Design review of the part built by this model. Coordinates are the model's own, in mm. Face numbers are marked on the shaded views. A direction names the side the tool comes from. Coordinates: 2 decimals unless noted, no trailing zeros. Write each loop counter-clockwise with the first axis right and the second up, starting at its lowest first coordinate (ties: lowest second). Pieces come first, ordered by that corner, then holes. Notation, with made-up numbers: (-26, 66.5) - (12, 66.5) arc R5 cw to (12, 75.5) - close; hole circle Ø7 at (68.25, 77). An arc over 180 degrees is marked (long way). One line per item, written item: value.
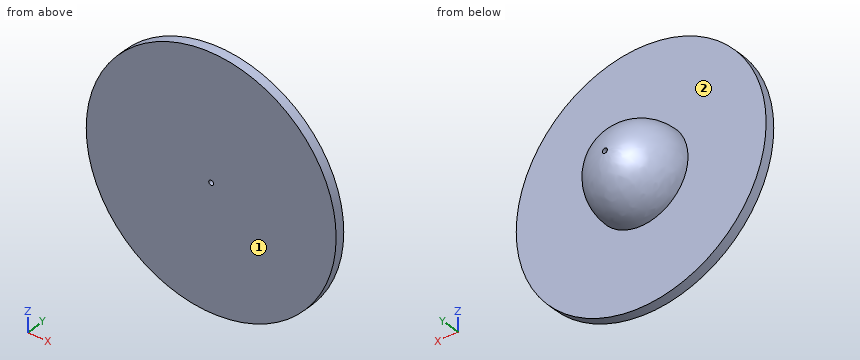
Autodesk Inventor part; units mm, degrees
ref_plane "YZ Plane" through (0, 0, 0) normal (1, 0, 0) x (0, 1, 0)
ref_plane "XZ Plane" through (0, 0, 0) normal (0, 1, 0) x (-1, 0, 0)
ref_plane "XY Plane" through (0, 0, 0) normal (0, 0, 1) x (1, 0, 0)
sketch "Sketch1" plane through (0, 0, 0) normal (0, 1, 0) x (-1, 0, 0)
  circle A0 centre (0, 0) radius 25.4
  dimension "d0" = 50.8
extrude "Extrusion1" add sketch "Sketch1" along normal blind 2
sketch "Sketch3" plane through (0, 0, 0) normal (0, 0, 1) x (1, 0, 0)
  line L0 (-25.4, 0) -> (25.4, 0)
  line L1 (25.4, 2) -> (-25.4, 2)
  line L2 (0, 2) -> (0, 13.4486)
  arc A0 (9.3127, 0) -> (9.525, 2) centre (0, 2) ccw
  arc A1 (0, 11.525) -> (-9.3127, 0) centre (0, 2) ccw
  line L3 (0, 2) -> (-9.525, 2)
  point P0 (0, 0)
revolve "Revolution1" add sketch "Sketch3" angle 360 about axis through (0, 2, 0) along (0, 1, 0) contours A1 L2 L1
sketch "Sketch2" plane through (0, 2, 0) normal (0, 1, 0) x (1, 0, 0)
  circle A0 centre (0, 0) radius 25.4
  circle A1 centre (0, 0) radius 0.5
  dimension "d3" = 1
extrude "Extrusion2" cut sketch "Sketch2" along normal through all both and the other way through all contours A1
properties part number "flower"
1. For the marked faces 1 and 2, list the 3-axis set-ups (+Z, -Z, +X, -X, +Y, -Y) from which the entire face can be reached by the end or side of a thin tool; tool diameter is ignored.
Answer block:
face 1: +Z, -Z, +X, -X, -Y
face 2: +Y
2. Insertion check: pin 1 Ø2 at (y, z) = (5.5, 8) entering from +X; pin 2 Ø5 at (x, y) = (4.5, 9) entering from +Z; pin 3 Ø2 at (x, z) = (14.5, -9) entering from +Y. Each pin has a flat end and moves straight along its axis. Give the tip position at first contact, or say it passes through.
Answer block:
pin 1: stops at x = 5.56
pin 2: stops at z = 7.54
pin 3: stops at y = 2
3. Consider section B-B, the plane x = -21.5. Write out the cut boundary in (y, z).
Answer block:
outline: (0, -13.52) - (2, -13.52) - (2, 13.52) - (0, 13.52) - close
4. Consider section A-A, the plane z = -12.5. Write out the cut boundary in (x, y).
Answer block:
outline: (-22.11, 0) - (22.11, 0) - (22.11, 2) - (-22.11, 2) - close
5. Wall thickness on line 1 along Z through (x, y) = (0, 1.15); line 2 along Y through (x, z) = (15.5, -5.5); line 3 along X through (y, z) = (4.75, 0): over which ranges is each line inside the solid? List them lowest first.
Answer block:
line 1: z = -25.4 to -0.5, 0.5 to 25.4
line 2: y = 0 to 2
line 3: x = -9.12 to -0.5, 0.5 to 9.12
